For this review, take the finished solid that the model builds, in its own axes (mm). Round coordinates to 2 decimals unless told otherwise and drop trailing zeros. Order: outer loops, then holes, each group sorted by start corner. A loop starts at its lowest first (then second) coordinate and runs counter-clockwise, first axis right, second up. Notation, with made-up numbers: M 26,88.25 L 79,88.25 A16 cw 79,106.25 Z; hole C 23.25,-29.5 d2. An arc over 180 degrees is marked long. Use a Markdown table: item, result.
from build123d import *

# Parameters (mm, degrees)
SKETCH1_W           = 83.28
SKETCH1_H           = 30
BOSS_EXTRUDE1_DEPTH = 1
CUT_EXTRUDE2_DEPTH  = 45.270640384


with BuildPart() as part:
    # Sketch1 → Boss-Extrude1 (new body)
    with BuildSketch(Plane(origin=(0, 0, 0), x_dir=(0, 0, -1), z_dir=(1, 0, 0))):
        Rectangle(SKETCH1_W, SKETCH1_H)
    extrude(amount=BOSS_EXTRUDE1_DEPTH)

    # Sketch3 → Cut-Extrude2 (cut, through all)
    with BuildSketch(Plane(origin=(1, 0, 0), x_dir=(0, 0, -1), z_dir=(1, 0, 0))):
        with BuildLine():
            Line((4.64, 15), (4.64, 3))
            ThreePointArc((4.64, 3), (8.64, 7), (12.64, 3))
            Line((12.64, 3), (12.64, 15))
            Line((12.64, 15), (4.64, 15))
        make_face()
        with BuildLine():
            ThreePointArc((12.64, 3), (8.64, 7), (4.64, 3))
            Line((4.64, 3), (12.64, 3))
        make_face()
        with BuildLine():
            Line((12.64, 3), (4.64, 3))
            ThreePointArc((4.64, 3), (8.64, -1), (12.64, 3))
        make_face()
    extrude(amount=-CUT_EXTRUDE2_DEPTH, mode=Mode.SUBTRACT)


solid = part.part
Q1. Add section A-A (y = 6.5). Write out the cut boundary in (x, z), then the cut area to 3 significant figures.
Determined:
| item | result |
|---|---|
| outline | M 0,-41.64 L 1,-41.64 L 1,-12.64 L 0,-12.64 Z; M 0,-4.64 L 1,-4.64 L 1,41.64 L 0,41.64 Z |
| area | 75.3 mm^2 |
Q2. Wall thickness on line 1 along Z through (x, y) = (0.7, 12.25); line 2 along Z through (x, y) = (0.8, 2); line 3 along Y through (x, z) = (0.55, -8): over which ranges is each line inside the solid? List them lowest first. Write a range as [from, to].
Determined:
| item | result |
|---|---|
| line 1 | z = [-41.64, -12.64], [-4.64, 41.64] |
| line 2 | z = [-41.64, -12.51], [-4.77, 41.64] |
| line 3 | y = [-15, -0.95] |
Q3. Draft analysis for pull direction Z (two halves, no side actions). For faces 1 (the cylindrical face through (0.5, -1, -8.6)), 2 (the flat face through (1, 0, 1)), state which applies: pulls with the +Z half, pulls with the -Z half, needs draft (parallel to the pull), parting line crosses it, or undercut.
Determined:
| item | result |
|---|---|
| face 1 | undercut |
| face 2 | needs draft |
Q4. Add section C-C (z = -8.64). Write out the cut boundary in (x, y).
Determined:
| item | result |
|---|---|
| outline | M 0,-15 L 1,-15 L 1,-1 L 0,-1 Z |
Q5. Add section B-B (x = 0.65). Write out the cut boundary in (y, z), then the cut area to 3 significant figures.
Determined:
| item | result |
|---|---|
| outline | M -15,-41.64 L 15,-41.64 L 15,-12.64 L 3,-12.64 A4 cw 3,-4.64 L 15,-4.64 L 15,41.64 L -15,41.64 Z |
| area | 2,380 mm^2 |
